```python
from build123d import *

# Parameters (mm, degrees)
SKETCH_1_R          = 16.5
EXTRUDE_1_DEPTH     = 6
SKETCH_2_R          = 4.25
CUT_EXTRUDE_1_DEPTH = 25.093567606
SKETCH_3_R          = 0.6
CUT_EXTRUDE_2_DEPTH = 3
SKETCH_4_R          = 16.5
SKETCH_4_R_2        = 5.5
EXTRUDE_2_DEPTH     = 10
SKETCH_5_R          = 5.5
EXTRUDE_3_DEPTH     = 122
SKETCH_6_W          = 29
SKETCH_6_H          = 40
SKETCH_6_W_2        = 10
SKETCH_6_H_2        = 20
CUT_EXTRUDE_3_DEPTH = 3
SKETCH_7_W          = 4
SKETCH_7_H          = 40
CUT_EXTRUDE_4_DEPTH = 5
SKETCH_8_R          = 0.4
CUT_EXTRUDE_5_DEPTH = 2
SKETCH_9_R          = 0.6
CUT_EXTRUDE_6_DEPTH = 2
SKETCH_10_R         = 0.6
CUT_EXTRUDE_7_DEPTH = 3
SKETCH_11_R         = 0.6
CUT_EXTRUDE_8_DEPTH = 3
SKETCH_12_R         = 1.5
CUT_EXTRUDE_9_DEPTH = 40


with BuildPart() as part:
    # 草图1 → 凸台-拉伸1 (new body)
    with BuildSketch(Plane(origin=(0, 0, 0), x_dir=(1, 0, 0), z_dir=(0, 1, 0))):
        with Locations(Location((0, 0, 0), (0, 0, 270))):
            Circle(SKETCH_1_R)
    extrude(amount=EXTRUDE_1_DEPTH)

    # 草图2 → 切除-拉伸1 (cut, through all)
    with BuildSketch(Plane(origin=(0, 6, 0), x_dir=(1, 0, 0), z_dir=(0, 1, 0))):
        with Locations(Location((0, -8, 0), (0, 0, 270))):
            Circle(SKETCH_2_R)
    extrude(amount=-CUT_EXTRUDE_1_DEPTH, mode=Mode.SUBTRACT)

    # 草图3 → 切除-拉伸2 (cut)
    with BuildSketch(Plane.XZ):
        with Locations(Location((-8.485281374, 8.485281374, 0), (0, 0, 270))):
            Circle(SKETCH_3_R)
        with Locations(Location((8.485281374, 8.485281374, 0), (0, 0, 270))):
            Circle(SKETCH_3_R)
        with Locations(Location((8.485281374, -8.485281374, 0), (0, 0, 270))):
            Circle(SKETCH_3_R)
        with Locations(Location((-8.485281374, -8.485281374, 0), (0, 0, 270))):
            Circle(SKETCH_3_R)
    extrude(amount=-CUT_EXTRUDE_2_DEPTH, mode=Mode.SUBTRACT)

    # 草图4 → 凸台-拉伸2 (add)
    with BuildSketch(Plane(origin=(0, 6, 0), x_dir=(1, 0, 0), z_dir=(0, 1, 0))):
        with Locations(Location((0, 0, 0), (0, 0, 270))):
            Circle(SKETCH_4_R)
        with Locations(Location((0, -8, 0), (0, 0, 270))):
            Circle(SKETCH_4_R_2, mode=Mode.SUBTRACT)
    extrude(amount=EXTRUDE_2_DEPTH)

    # 草图5 → 凸台-拉伸3 (add)
    with BuildSketch(Plane(origin=(0, 16, 0), x_dir=(1, 0, 0), z_dir=(0, 1, 0))):
        with BuildLine():
            ThreePointArc((-16.5, 0), (0, -16.5), (16.5, 0))
            Line((16.5, 0), (-16.5, 0))
        make_face()
        with Locations(Location((0, -8, 0), (0, 0, 270))):
            Circle(SKETCH_5_R, mode=Mode.SUBTRACT)
    extrude(amount=EXTRUDE_3_DEPTH)

    # 草图6 → 切除-拉伸3 (cut)
    with BuildSketch(Plane(origin=(0, 0, 0), x_dir=(-1, 0, 0), z_dir=(0, 0, -1))):
        with Locations((0, 118)):
            Rectangle(SKETCH_6_W, SKETCH_6_H)
        with Locations((0, 88)):
            Rectangle(SKETCH_6_W_2, SKETCH_6_H_2)
    extrude(amount=-CUT_EXTRUDE_3_DEPTH, mode=Mode.SUBTRACT)

    # 草图7 → 切除-拉伸4 (cut)
    with BuildSketch(Plane(origin=(0, 0, 3), x_dir=(-1, 0, 0), z_dir=(0, 0, -1))):
        with Locations((9.1, 118)):
            Rectangle(SKETCH_7_W, SKETCH_7_H)
        with Locations((-9.1, 118)):
            Rectangle(SKETCH_7_W, SKETCH_7_H)
    extrude(amount=-CUT_EXTRUDE_4_DEPTH, mode=Mode.SUBTRACT)

    # 草图8 → 切除-拉伸5 (cut)
    with BuildSketch(Plane(origin=(0, 0, 3), x_dir=(-1, 0, 0), z_dir=(0, 0, -1))):
        with Locations((-12.8, 133)):
            Circle(SKETCH_8_R)
        with Locations((-12.8, 110)):
            Circle(SKETCH_8_R)
        with Locations((12.8, 133)):
            Circle(SKETCH_8_R)
        with Locations((12.8, 110)):
            Circle(SKETCH_8_R)
    extrude(amount=-CUT_EXTRUDE_5_DEPTH, mode=Mode.SUBTRACT)

    # 草图9 → 切除-拉伸6 (cut)
    with BuildSketch(Plane(origin=(0, 0, 0), x_dir=(-1, 0, 0), z_dir=(0, 0, -1))):
        with Locations((0, 67)):
            Circle(SKETCH_9_R)
        with Locations((0, 47)):
            Circle(SKETCH_9_R)
    extrude(amount=-CUT_EXTRUDE_6_DEPTH, mode=Mode.SUBTRACT)

    # 草图10 → 切除-拉伸7 (cut)
    with BuildSketch(Plane(origin=(0, 0, 0), x_dir=(-1, 0, 0), z_dir=(0, 0, -1))):
        with Locations((-8.5, 87)):
            Circle(SKETCH_10_R)
        with Locations((8.5, 87)):
            Circle(SKETCH_10_R)
        with Locations((8.5, 27)):
            Circle(SKETCH_10_R)
        with Locations((-8.5, 27)):
            Circle(SKETCH_10_R)
    extrude(amount=-CUT_EXTRUDE_7_DEPTH, mode=Mode.SUBTRACT)

    # 草图11 → 切除-拉伸8 (cut)
    with BuildSketch(Plane(origin=(0, 138, 0), x_dir=(1, 0, 0), z_dir=(0, 1, 0))):
        with Locations(Location((7.743281891, -11.058552598, 0), (0, 0, 270))):
            Circle(SKETCH_11_R)
        with Locations(Location((-7.743281891, -11.058552598, 0), (0, 0, 270))):
            Circle(SKETCH_11_R)
    extrude(amount=-CUT_EXTRUDE_8_DEPTH, mode=Mode.SUBTRACT)

    # 草图12 → 切除-拉伸9 (cut)
    with BuildSketch(Plane(origin=(0, 0, 0), x_dir=(-1, 0, 0), z_dir=(0, -1, 0))):
        with Locations(Location((0, 0, 0), (0, 0, 90))):
            Circle(SKETCH_12_R)
    extrude(amount=-CUT_EXTRUDE_9_DEPTH, mode=Mode.SUBTRACT)


solid = part.part
```
Read the model definition and answer for the solid it produces. Units are mm, in the model's axes. A direction names the side the tool comes from. Coordinates: 2 decimals unless noted, no trailing zeros. Write each loop counter-clockwise with the first axis right and the second up, starting at its lowest first coordinate (ties: lowest second). Pieces come first, ordered by that corner, then holes. Notation, with made-up numbers: (-17, -19) -> (-8, -19) arc R5 ccw to (-8, -10) -> close; hole circle Ø2 at (81.5, 87). An arc over 180 degrees is marked (long way). Answer as a JSON object with one key per item and string values.
Q1. The part is cut by section A-A on y = 108. Give the vertices of the cut face in (x, z), then the cut area to 3 significant figures.
The answers:
{"outline": "(-16.5, 0) -> (-14.5, 0) -> (-14.5, 3) -> (-11.1, 3) -> (-11.1, 8) -> (-7.1, 8) -> (-7.1, 3) -> (-2.29, 3) arc R5.5 cw (long way) to (2.29, 3) -> (7.1, 3) -> (7.1, 8) -> (11.1, 8) -> (11.1, 3) -> (14.5, 3) -> (14.5, 0) -> (16.5, 0) arc R16.5 ccw to start", "area": "207 mm2"}
Q2. Consider line 1 (Y direction, x = 12.8, z = 3.45); line 2 (X direction, y = 110, z = 4.65); line 3 (X direction, y = 87, z = 1.15). Determine where each line is inside the solid, lowest interval first. Write a range as [from, to].
The answers:
{"line 1": "y = [0, 109.6], [110.4, 132.6], [133.4, 138]", "line 2": "x = [-15.83, -13.2], [-12.4, -11.1], [-7.1, -4.36], [4.36, 7.1], [11.1, 12.4], [13.2, 15.83]", "line 3": "x = [-16.46, -9.1], [-7.9, -5], [5, 7.9], [9.1, 16.46]"}
Q3. The part is cut by section D-D on z = -10.5. Give the vertices of the cut face in (x, y).
The answers:
{"outline": "(-12.73, 0) -> (12.73, 0) -> (12.73, 16) -> (-12.73, 16) -> close"}
Q4. The part is cut by section C-C on y = 13.5. Give the vertices of the cut face in (x, z).
The answers:
{"outline": "circle Ø33 at (0, 0); hole circle Ø11 at (0, 8); hole circle Ø3 at (0, 0)"}
Q5. Flat-ended cylindrical pins translate along their axes: pin 1 Ø1 at (x, y) = (-8.5, 27) entering from -Z; pin 2 Ø4 at (x, y) = (-8.5, 62) entering from -Z; pin 3 Ø1.5 at (y, z) = (63, 1) entering from -X. Find the tip coordinate at first contact, or state that the pin passes through.
The answers:
{"pin 1": "stops at z = 3", "pin 2": "stops at z = 0", "pin 3": "stops at x = -16.5"}
Q6. Determine the mould class of faces 1 (the flat face through (-3, 0, 0)), 2 (the flat face through (10, 98, 3)), 3 (the flat face through (-5, 115, 3)) for opening direction Y: pulls with the +Y half, pulls with the -Y half, needs draft (parallel to the pull), parting line crosses it, or undercut.
The answers:
{"face 1": "pulls with the -Y half", "face 2": "pulls with the +Y half", "face 3": "needs draft"}
Q7. The part is cut by section B-B on y = 69. Give the vertices of the cut face in (x, z), then the cut area to 3 significant figures.
The answers:
{"outline": "(-16.5, 0) -> (16.5, 0) arc R16.5 ccw to start; hole circle Ø11 at (0, 8)", "area": "333 mm2"}
Q8. A tool of negligible diameter and unlimited length cuts with its end or side. For faces 4 (the flat face through (0, 78, 1)), 5 (the flat face through (0, 16, -7)), 6 (the flat face through (1, 138, 14)), 7 (the cylindrical face through (0.07, 15.28, 1.5)), from which of +Z, -Z, +X, -X, +Y, -Y can it reach the whole face along a straight path? Write none if from no direction.
The answers:
{"face 4": "-Z, +Y", "face 5": "-Z, +X, -X, +Y", "face 6": "+Z, -Z, +X, -X, +Y", "face 7": "-Y"}
